Model file for the job. Use its own axes, mm. A direction names the side the tool comes from. Give positions to 0.01 mm unless a question says otherwise; leave off trailing zeros. Order: outer loops, then holes, each group sorted by start corner. A loop starts at its lowest first (then second) coordinate and runs counter-clockwise, first axis right, second up. Notation, with made-up numbers: (85, -22) -> (135, -22) arc R14 ccw to (135, -17) -> close; hole circle Ø1 at (-17.5, -40). An arc over 180 degrees is marked (long way). Use CSV: the item, a comma, the result in double quotes. Start each with the question number.
1. Cut at C-C on x = 25. Give the number of separate pieces and of enclosed holes in the cut face, then the cut area to 3 significant figures.
2. Cut at B-B on y = -51.5. List the corners of the cut face in (x, z), then the cut area to 3 significant figures.
3. Cut at A-A on x = -118.3. List the corners of the cut face in (y, z), then the cut area to 3 significant figures.
4. Drop flat-ended pins along their axis: pin 1 (3.5 mm diameter, centred on x = -118.3, y = -25, fed in from +Z); pin 2 (1 mm diameter, centred on x = 22.5, y = -25.5, fed in from +Z). Give the stop position or say it passes through.
5. Pull direction X, two halves, no side cores. Call faces 4 (the flat face through (-117, 27, 10)), 5 (the flat face through (-158.352, -50, 6)), 6 (the flat face through (-58, -78.354, 8)): released by +X, released by -X, zero draft, split by the parting line, or undercut.
6. Wall check: line 1 (Y direction, x = -107.5, z = 1.5); line 2 (X direction, y = -6.5, z = 8.75); line 3 (X direction, y = -30, z = 2.5). Give the ranges that are in metal, low to high. Write a range as from..to.
7. 3-axis set-ups, long thin cutter, end or side, ignore diameter. For faces 1 (the flat face through (25.9, 27.1, 10)), 2 (the flat face through (-113, -29.948, 6)), 3 (the flat face through (0, 20, 7)): which of +Z, -Z, +X, -X, +Y, -Y reach the whole face in a straight line?
Autodesk Inventor part; units mm, degrees
ref_plane "YZ Plane" through (0, 0, 0) normal (1, 0, 0) x (0, 1, 0)
ref_plane "XZ Plane" through (0, 0, 0) normal (0, 1, 0) x (-1, 0, 0)
ref_plane "XY Plane" through (0, 0, 0) normal (0, 0, 1) x (1, 0, 0)
ref_plane "Work Plane1" through (0, 0, 0) normal (0, 0, 1) x (1, 0, 0)
ref_plane "Work Plane2" through (0, 0, 0) normal (0, 0, 1) x (1, 0, 0)
sketch "Sketch3" plane through (0, 0, 0) normal (0, 0, 1) x (1, 0, 0)
  circle A0 centre (0, 25) radius 1.95 construction
  circle A1 centre (-25, 0) radius 1.95 construction
  circle A2 centre (-25, -25) radius 1.95 construction
  circle A3 centre (25, 25) radius 1.95 construction
  circle A4 centre (25, -25) radius 1.95 construction
  circle A5 centre (-25, 25) radius 1.95 construction
  circle A6 centre (25, 0) radius 1.95 construction
  circle A7 centre (0, -25) radius 1.95 construction
  line L0 (-28, 30) -> (-30, 28) construction
  line L1 (-30, 28) -> (-30, -28) construction
  line L2 (-30, -28) -> (-28, -30) construction
  line L3 (-28, -30) -> (28, -30) construction
  line L4 (28, -30) -> (30, -28) construction
  line L5 (30, -28) -> (30, 28) construction
  line L6 (30, 28) -> (28, 30) construction
  line L7 (28, 30) -> (-28, 30) construction
  line L8 (30.0525, 30.0525) -> (-59.15, 30.0525)
  line L9 (-59.15, 30.0525) -> (-59.15, -29.9475)
  line L10 (-59.15, -29.9475) -> (30.0525, -29.9475)
  line L11 (30.0525, -29.9475) -> (30.0525, 30.0525)
  line L12 (-59.15, -29.9475) -> (-49.9475, -29.9475)
  line L13 (-49.9475, -29.9475) -> (-49.9475, -69.9475)
  line L14 (-49.9475, -69.9475) -> (-59.15, -69.9475)
  line L15 (-59.15, -69.9475) -> (-59.15, -29.9475)
  circle A8 centre (-59.15, -56.5073) radius 2.9125 construction
  point P0 (0, 0)
  dimension "d6" = 60
  dimension "d8" = 40
extrude "Extrusion2" add sketch "Sketch3" along normal blind 12
sketch "Sketch4" plane through (0, 0, 12) normal (0, 0, 1) x (1, 0, 0)
  line L0 (-59.15, 30.0525) -> (-59.15, -69.9475)
  line L1 (-59.15, -69.9475) -> (-49.9475, -69.9475)
  line L2 (-49.9475, -69.9475) -> (-49.9475, -29.9475)
  line L3 (-49.9475, -29.9475) -> (30.0525, -29.9475)
  line L4 (30.0525, -29.9475) -> (30.0525, 30.0525)
  line L5 (30.0525, 30.0525) -> (-59.15, 30.0525)
  line L6 (-49.9475, -69.9475) -> (30.0525, -69.9475)
  line L7 (30.0525, -69.9475) -> (30.0525, -29.9475)
  line L8 (30.0525, -29.9475) -> (-49.9475, -29.9475)
  line L9 (-49.9475, -29.9475) -> (-49.9475, -69.9475)
  point P0 (0, 0)
extrude "Extrusion3" add sketch "Sketch4" along normal blind 3
sketch "Sketch5" plane through (0, 0, 15) normal (0, 0, 1) x (1, 0, 0)
  line L0 (-59.15, -69.9475) -> (30.0525, -69.9475)
  line L1 (30.0525, -69.9475) -> (30.0525, 30.0525)
  line L2 (30.0525, 30.0525) -> (-59.15, 30.0525)
  line L3 (-59.15, 30.0525) -> (-59.15, -69.9475)
  line L4 (-59.15, -69.9475) -> (-49.9475, -69.9475)
  line L5 (-59.15, -69.9475) -> (50.85, -69.9475)
  line L6 (50.85, -69.9475) -> (50.85, -78.3535)
  line L7 (50.85, -78.3535) -> (-59.15, -78.3535)
  line L8 (-59.15, -78.3535) -> (-59.15, -69.9475)
  line L9 (50.85, -78.3535) -> (54.85, -78.3535)
  line L10 (54.85, -78.3535) -> (54.85, -24.0007)
  line L11 (54.85, -24.0007) -> (50.85, -24.0007)
  line L12 (50.85, -24.0007) -> (50.85, -78.3535)
  point P0 (0, 0)
  dimension "d13" = 110
  dimension "d14" = 8.406
  dimension "d15" = 4
  dimension "d16" = 54.353
extrude "Extrusion4" add sketch "Sketch5" against normal up to surface (15 mm away) contours L0 L5 L6 L7 L8
sketch "Sketch6" plane through (0, 0, 15) normal (0, 0, 1) x (1, 0, 0)
  line L0 (30.0525, -69.9475) -> (30.0525, 30.0525)
  line L1 (30.0525, 30.0525) -> (-59.15, 30.0525)
  line L2 (-59.15, 30.0525) -> (-59.15, -78.3535)
  line L3 (-59.15, -78.3535) -> (50.85, -78.3535)
  circle A0 centre (0, 25) radius 1.95
  circle A1 centre (-25, 0) radius 1.95
  circle A2 centre (-25, -25) radius 1.95
  circle A3 centre (25, 25) radius 1.95
  circle A4 centre (25, -25) radius 1.95
  circle A5 centre (-25, 25) radius 1.95
  circle A6 centre (25, 0) radius 1.95
  circle A7 centre (0, -25) radius 1.95
  line L4 (-28, 30) -> (-30, 28)
  line L5 (-30, 28) -> (-30, -28)
  line L6 (-30, -28) -> (-28, -30)
  line L7 (-28, -30) -> (28, -30)
  line L8 (28, -30) -> (30, -28)
  line L9 (30, -28) -> (30, 28)
  line L10 (30, 28) -> (28, 30)
  line L11 (28, 30) -> (-28, 30)
  line L12 (50.85, -78.3535) -> (50.85, -69.9475)
  line L13 (50.85, -69.9475) -> (30.0525, -69.9475)
  point P0 (0, 0)
hole "Hole1" at (25, 25, 15) at (0, 25, 15) at (-25, 25, 15) at (-25, 0, 15) at (-25, -25, 15) at (0, -25, 15) at (25, -25, 15) at (25, 0, 15) direction (0, 0, -1) diameter 4.2 end through all counterbore diameter 9 counterbore depth 5
sketch "Sketch7" plane through (30.0525, -29.9475, 0) normal (1, 0, 0) x (0, 0, -1)
  line L0 (-10, 34.4475) -> (-10, 25.4475)
  line L1 (0, 0) -> (0, 60)
  line L2 (0, 60) -> (-15, 60)
  line L3 (-15, -40) -> (-15, 60)
  line L4 (-12, -40) -> (-12, 0)
  line L5 (0, 0) -> (-12, 0)
  line L6 (-12, -40) -> (-15, -40)
  point P0 (0, 29.9475)
extrude "Extrusion5" add sketch "Sketch7" along normal blind 10
sketch "Sketch8" plane through (40.0525, -29.9475, 0) normal (1, 0, 0) x (0, 0, -1)
  line L0 (0, 0) -> (0, 60)
  line L1 (0, 60) -> (-15, 60)
  line L2 (-15, 60) -> (-15, -40)
  line L3 (-12, -40) -> (-12, 0)
  line L4 (-12, 0) -> (0, 0)
  line L5 (0, 0) -> (-12, 0)
  line L6 (-12, 0) -> (-12, -40)
  line L7 (-12, -40) -> (0, -40)
  line L8 (0, -40) -> (0, 0)
  line L9 (-12, -40) -> (-15, -40)
  point P0 (0, 29.9475)
extrude "Extrusion6" add sketch "Sketch8" along normal up to surface (10.7975 mm away)
sketch "Sketch10" plane through (0, 0, 0) normal (0, 0, -1) x (-1, 0, 0)
  line L0 (49.9475, -29.9475) -> (-40.0525, -29.9475) construction
  line L1 (49.9475, -69.9475) -> (49.9475, -29.9475) construction
  line L2 (49.9475, -69.9475) -> (-40.0525, -69.9475) construction
  line L3 (-40.0525, -69.9475) -> (-40.0525, -29.9475) construction
  circle A0 centre (-25, -25) radius 2.1 construction
  circle A1 centre (25, -25) radius 2.1 construction
  circle A2 centre (25, 25) radius 2.1 construction
  circle A3 centre (-25, 25) radius 2.1 construction
  circle A4 centre (0, 25) radius 2.1 construction
  circle A5 centre (25, 0) radius 2.1 construction
  circle A6 centre (0, -25) radius 2.1 construction
  circle A7 centre (-25, 0) radius 2.1 construction
  line L4 (-50.85, 30.0525) -> (59.15, 30.0525) construction
  line L5 (-50.85, -78.3535) -> (59.15, -78.3535) construction
  line L6 (59.15, 30.0525) -> (59.15, -78.3535) construction
  line L7 (39, -67) -> (34, -67) construction
  line L8 (34, -71) -> (34, -67) construction
  line L9 (34, -71) -> (39, -71) construction
  line L10 (39, -67) -> (39, -71) construction
  line L11 (28.1949, -69.9475) -> (49.9475, -69.9475)
  line L12 (49.9475, -69.9475) -> (49.9475, -73.7985)
  line L13 (49.9475, -73.7985) -> (28.1949, -73.7985)
  line L14 (28.1949, -73.7985) -> (28.1949, -69.9475)
  line L15 (-50.85, 30.0525) -> (-50.85, -78.3535)
  point P0 (0, 0)
extrude "Extrusion8" cut sketch "Sketch10" against normal up to surface (12 mm away)
sketch "Sketch15" plane through (0, 0, 0) normal (0, 0, -1) x (-1, 0, 0)
  circle A0 centre (0, 0) radius 7.5
  line L0 (20, -20) -> (-20, -20)
  line L1 (-20, -20) -> (-20, 20)
  line L2 (-20, 20) -> (20, 20)
  line L3 (20, 20) -> (20, -20)
  line L4 (20, -20) -> (-20, 20) construction
  line L5 (-20, -20) -> (20, 20) construction
  point P0 (0, 0)
  dimension "d52" = 40
  dimension "d53" = 40
extrude "Extrusion10" cut sketch "Sketch15" against normal through all contours A0 | L0 L1 L2 L3
mirror "Mirror2" about plane through (-59.15, -29.9475, 0) normal (-1, 0, 0) of "Extrusion2", "Extrusion3", "Extrusion4", "Hole1", "Extrusion5", "Extrusion6", "Extrusion8", "Extrusion10"
sketch "Sketch20" plane through (0, 0, 0) normal (0, 0, -1) x (-1, 0, 0)
  circle A0 centre (59.15, -56.5073) radius 2.9125
  line L0 (14, -48.5) -> (-39, -48.5)
  line L1 (14, -53.5) -> (-39, -53.5)
  line L2 (-21.1695, -50.8251) -> (110.767, -50.8251)
  line L3 (52.1305, -46.7848) -> (66.1268, -46.7848)
  line L4 (66.1268, -46.7848) -> (59.1286, -58.9059)
  line L5 (59.1286, -58.9059) -> (52.1305, -46.7848)
  point P0 (0, 0)
  point P1 (59.1286, -50.8251)
  dimension "d75" = 180
hole "Hole6" at (-52.1305, -46.7848, 0) at (-66.1268, -46.7848, 0) at (-59.1286, -58.9059, 0) direction (0, 0, 1) diameter 2.8 end through all
sketch "Sketch21" plane through (0, 0, 0) normal (0, 0, -1) x (-1, 0, 0)
  circle A0 centre (66.1268, -46.7848) radius 1.4
  circle A1 centre (52.1305, -46.7848) radius 1.4
  circle A2 centre (59.1286, -58.9059) radius 1.4
  line L0 (169.15, 30.0525) -> (169.15, -78.3535)
  line L1 (-50.85, 30.0525) -> (169.15, 30.0525)
  line L2 (-50.85, 30.0525) -> (-50.85, -78.3535)
  line L3 (-50.85, -78.3535) -> (169.15, -78.3535)
  circle A3 centre (-25, 0) radius 2.1
  circle A4 centre (0, -25) radius 2.1
  circle A5 centre (25, 0) radius 2.1
  circle A6 centre (0, 25) radius 2.1
  circle A7 centre (-25, 25) radius 2.1
  circle A8 centre (25, 25) radius 2.1
  circle A9 centre (25, -25) radius 2.1
  circle A10 centre (-25, -25) radius 2.1
  line L4 (28.1949, -73.7985) -> (28.1949, -69.9475)
  line L5 (28.1949, -69.9475) -> (-40.0525, -69.9475)
  line L6 (-40.0525, -69.9475) -> (-40.0525, -29.9475)
  line L7 (49.9475, -29.9475) -> (-40.0525, -29.9475)
  line L8 (49.9475, -29.9475) -> (49.9475, -73.7985)
  line L9 (49.9475, -73.7985) -> (28.1949, -73.7985)
  line L10 (20, 20) -> (20, -20)
  line L11 (20, -20) -> (-20, -20)
  line L12 (-20, -20) -> (-20, 20)
  line L13 (-20, 20) -> (20, 20)
  circle A11 centre (93.3, -25) radius 2.1
  circle A12 centre (93.3, 25) radius 2.1
  circle A13 centre (143.3, 25) radius 2.1
  circle A14 centre (118.3, 25) radius 2.1
  circle A15 centre (93.3, 0) radius 2.1
  circle A16 centre (118.3, -25) radius 2.1
  circle A17 centre (143.3, 0) radius 2.1
  circle A18 centre (143.3, -25) radius 2.1
  line L14 (90.1051, -69.9475) -> (90.1051, -73.7985)
  line L15 (90.1051, -73.7985) -> (68.3525, -73.7985)
  line L16 (68.3525, -73.7985) -> (68.3525, -29.9475)
  line L17 (68.3525, -29.9475) -> (158.3525, -29.9475)
  line L18 (158.3525, -69.9475) -> (158.3525, -29.9475)
  line L19 (90.1051, -69.9475) -> (158.3525, -69.9475)
  line L20 (138.3, 20) -> (138.3, -20)
  line L21 (138.3, -20) -> (98.3, -20)
  line L22 (98.3, -20) -> (98.3, 20)
  line L23 (98.3, 20) -> (138.3, 20)
  line L24 (39.15, 20) -> (79.15, 20)
  line L25 (79.15, 20) -> (79.15, -20)
  line L26 (79.15, -20) -> (39.15, -20)
  line L27 (39.15, -20) -> (39.15, 20)
  line L28 (39.15, 20) -> (79.15, -20) construction
  line L29 (79.15, 20) -> (39.15, -20) construction
  point P0 (0, 0)
  point P1 (59.15, 0)
  dimension "d83" = 40
  dimension "d84" = 40
extrude "Extrusion13" cut sketch "Sketch21" against normal through all contours L24 L25 L26 L27
properties part number "10_Baseplate_Axiotech_mono"
Verdict:
1,separate pieces,"4"
1,enclosed holes,"0"
1,area,"885 mm^2"
2,outline,"(-169.15, 0) -> (-158.35, 0) -> (-158.35, 12) -> (-68.35, 12) -> (-68.35, 0) -> (-49.95, 0) -> (-49.95, 12) -> (40.05, 12) -> (40.05, 0) -> (50.85, 0) -> (50.85, 15) -> (-169.15, 15) -> close"
2,area,"1,140 mm^2"
3,outline,"(-78.35, 0) -> (-69.95, 0) -> (-69.95, 12) -> (-29.95, 12) -> (-29.95, 0) -> (-27.1, 0) -> (-27.1, 10) -> (-29.5, 10) -> (-29.5, 15) -> (-78.35, 15) -> close; (-22.9, 0) -> (-20, 0) -> (-20, 15) -> (-20.5, 15) -> (-20.5, 10) -> (-22.9, 10) -> close; (20, 0) -> (22.9, 0) -> (22.9, 10) -> (20.5, 10) -> (20.5, 15) -> (20, 15) -> close; (27.1, 0) -> (30.05, 0) -> (30.05, 15) -> (29.5, 15) -> (29.5, 10) -> (27.1, 10) -> close"
3,area,"372 mm^2"
4,pin 1,"through"
4,pin 2,"z = 10"
5,face 4,"undercut"
5,face 5,"undercut"
5,face 6,"zero draft"
6,line 1,"-78.35..-69.95, -29.95..-20, 20..30.05"
6,line 2,"-169.15..-138.3, -98.3..-79.15, -39.15..-20, 20..50.85"
6,line 3,"-169.15..-158.35, -68.35..-49.95, 40.05..50.85"
7,face 1,"+Z"
7,face 2,"-Z"
7,face 3,"+Z, -Z"
